```python
from build123d import *

# Parameters (mm, degrees)
F1_DEPTH = 500
F3_DEPTH = 1
F4_R     = 90
F5_DEPTH = 1
F6_R     = 35
F7_DEPTH = 1
F8_R     = 7.5
F9_DEPTH = 25


with BuildPart() as f1:
    # F0 (on Top) → F1 (new body)
    with BuildSketch(Plane.XY):
        with BuildLine():
            Line((200, 15), (0, 15))
            ThreePointArc((0, 15), (-15, 0), (0, -15))
            Line((0, -15), (200, -15))
            ThreePointArc((200, -15), (215, 0), (200, 15))
        make_face()
    extrude(amount=F1_DEPTH)

    # F2 (on face) → F3 (cut)
    with BuildSketch(Plane.XZ.offset(15)):
        with BuildLine():
            Line((180, 490), (20, 490))
            ThreePointArc((20, 490), (12.928932, 487.071068), (10, 480))
            Line((10, 480), (10, 350))
            ThreePointArc((10, 350), (12.928932, 342.928932), (20, 340))
            Line((20, 340), (180, 340))
            ThreePointArc((180, 340), (187.071068, 342.928932), (190, 350))
            Line((190, 350), (190, 480))
            ThreePointArc((190, 480), (187.071068, 487.071068), (180, 490))
        make_face()
    extrude(amount=-F3_DEPTH, mode=Mode.SUBTRACT)

    # F4 (on face) → F5 (cut)
    with BuildSketch(Plane.XZ.offset(15)):
        with Locations((100, 150)):
            Circle(F4_R)
    extrude(amount=-F5_DEPTH, mode=Mode.SUBTRACT)

    # F6 (on face) → F7 (cut)
    with BuildSketch(Plane.XZ.offset(14)):
        with Locations((100, 150)):
            Circle(F6_R)
    extrude(amount=-F7_DEPTH, mode=Mode.SUBTRACT)

    # F8 (on face) → F9 (cut)
    with BuildSketch(Plane.XY.offset(500)):
        with Locations((200, 0)):
            Circle(F8_R)
    extrude(amount=-F9_DEPTH, mode=Mode.SUBTRACT)


solid = f1.part
```
Work out the finished part from the listing and answer in its coordinate system (mm). A direction names the side the tool comes from. Coordinates: 2 decimals unless noted, no trailing zeros. Order: outer loops, then holes, each group sorted by start corner. A loop starts at its lowest first (then second) coordinate and runs counter-clockwise, first axis right, second up. Notation, with made-up numbers: (73, -17) - (98, -17) arc R9 ccw to (98, -9) - close; hole circle Ø7 at (76, -17.75). An arc over 180 degrees is marked (long way). Answer as a JSON object with one key per item and string values.
1. Find section A-A on z = 150. Determine the outline of the cut face in (x, y), plus the area to 3 significant figures.
Output values:
{"outline": "(0, -15) - (10, -15) - (10, -14) - (65, -14) - (65, -13) - (135, -13) - (135, -14) - (190, -14) - (190, -15) - (200, -15) arc R15 ccw to (200, 15) - (0, 15) arc R15 ccw to start", "area": "6,460 mm²"}
2. The mould has two halves that part along Y. Classify faces 1 (the face through (99, -15, 246)), 2 (the face through (215, 0, 246)), 3 (the face through (200, 0, 475)): +Y half, -Y half, draft (parallel to the pull), parting line (faces both ways), or undercut.
Output values:
{"face 1": "-Y half", "face 2": "parting line", "face 3": "undercut"}
3. Find section B-B on x = 101.5. Determine the outline of the cut face in (y, z).
Output values:
{"outline": "(-15, 0) - (15, 0) - (15, 500) - (-15, 500) - (-15, 490) - (-14, 490) - (-14, 340) - (-15, 340) - (-15, 239.99) - (-14, 239.99) - (-14, 184.97) - (-13, 184.97) - (-13, 115.03) - (-14, 115.03) - (-14, 60.01) - (-15, 60.01) - close"}
4. Each of these flat-tipped pins is pushed along its axis until it touches: P1, Ø5, axis at y = -9.5, z = 239, coming from the -X side; P2, Ø7.5, axis at x = 201, y = 1, coming from the +Z side; P3, Ø6, axis at y = -8.5, z = 393, coming from the -X side. Where does it stop, or does it pass through?
Output values:
{"P1": "stops at x = -13.27", "P2": "stops at z = 475", "P3": "stops at x = -13.96"}
5. A tool of negligible diameter and unlimited length cuts with its end or side. For faces 4 (the face through (100, -13, 150)), 5 (the face through (101, 15, 246)), 6 (the face through (206.93, -2.87, 487.68)), from which of +Z, -Z, +X, -X, +Y, -Y can it reach the whole face along a straight path? Write none if from no direction.
Output values:
{"face 4": "-Y", "face 5": "+Z, -Z, +X, -X, +Y", "face 6": "+Z"}
6. Consider line 1 (Y direction, x = 200, z = 488); line 2 (Z direction, x = 100, y = -14.2); line 3 (Z direction, x = 202.5, y = -6). Determine where each line is inside the solid, lowest interval first.
Output values:
{"line 1": "y = -15 to -7.5, 7.5 to 15", "line 2": "z = 0 to 60, 240 to 340, 490 to 500", "line 3": "z = 0 to 475"}
7. Find section C-C on z = 382. Determine the outline of the cut face in (x, y), plus the area to 3 significant figures.
Output values:
{"outline": "(0, -15) - (10, -15) - (10, -14) - (190, -14) - (190, -15) - (200, -15) arc R15 ccw to (200, 15) - (0, 15) arc R15 ccw to start", "area": "6,530 mm²"}
8. Find section D-D on x = 34.5. Determine the outline of the cut face in (y, z).
Output values:
{"outline": "(-15, 0) - (15, 0) - (15, 500) - (-15, 500) - (-15, 490) - (-14, 490) - (-14, 340) - (-15, 340) - (-15, 211.72) - (-14, 211.72) - (-14, 88.28) - (-15, 88.28) - close"}
